The model under review builds one solid part; all positions refer to its coordinate system, in mm. Face numbers are marked on the shaded views. Round coordinates to 2 decimals unless told otherwise and drop trailing zeros. Loops run counter-clockwise (first coordinate to the right, second up) from the corner with the lowest first, then second, coordinate; pieces in that order, holes last. Notation, with made-up numbers: M -6.5,24 L 5.5,24 A12 ccw 5.5,46 Z; hole C -11,48 d5. An arc over 180 degrees is marked long. Answer as a JSON object with one key per item and string values. Group by question number.
Item 1: Consider section C-C (x = -20). Give the boundary of the cut face in (y, z), and give its area (3 significant figures).
Item 2: Consider section B-B (y = 2.7). Give the boundary of the cut face in (x, z).
Item 3: To check wall thickness, follow line 1 (X direction, y = 1.55, z = -6.35); line 2 (X direction, y = 1.6, z = -7); line 3 (Z direction, x = -5.5, y = 4.35). State the ranges of each line that lie inside material, in increasing order.
Item 4: The part is to be moulded in two halves that separate along X. For the marked faces 1, 2 and 3, say which applies: +X half, -X half, draft (parallel to the pull), parting line (faces both ways), or undercut.
Item 5: Insertion check: P1, Ø6, axis at x = -6.5, z = -5.5, coming from the -Y side. The pin has a flat end and moves straight along its axis. Give the tip position at first contact, or say it passes through.
Item 6: Consider section D-D (z = -8.25). Give the boundary of the cut face in (x, y), and give its area (3 significant figures).
Item 7: Consider section A-A (z = -6.35). Give the boundary of the cut face in (x, y), and give its area (3 significant figures).
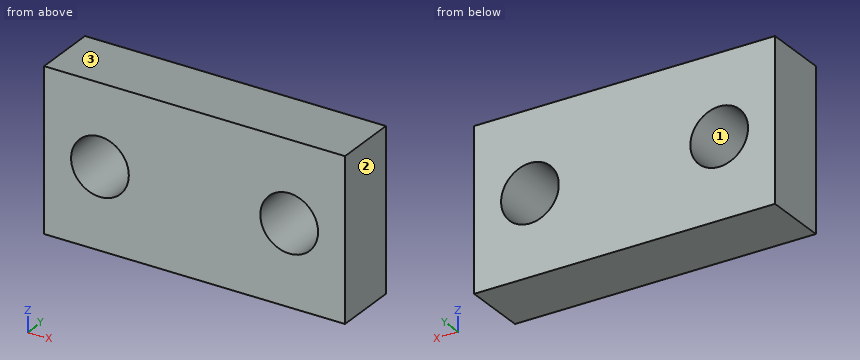
Autodesk Inventor part; units mm, degrees
ref_plane "YZ Plane" through (0, 0, 0) normal (1, 0, 0) x (0, 1, 0)
ref_plane "XZ Plane" through (0, 0, 0) normal (0, 1, 0) x (-1, 0, 0)
ref_plane "XY Plane" through (0, 0, 0) normal (0, 0, 1) x (1, 0, 0)
sketch "Spacer 2D" plane through (0, 0, 0) normal (0, 1, 0) x (-1, 0, 0)
  line L0 (12.4883, 0) -> (12.4883, -12.7) construction
  line L1 (24.4009, -12.7) -> (0.5757, -12.7)
  line L2 (0.5757, -12.7) -> (0.5757, 0)
  line L3 (0.5757, 0) -> (24.4009, 0)
  line L4 (24.4009, 0) -> (24.4009, -12.7)
  line L5 (24.4009, -12.7) -> (0.5757, 0) construction
  line L6 (0.5757, -12.7) -> (24.4009, 0) construction
  point P0 (0, 0)
  point P1 (12.4883, -6.35)
  dimension "d17" = 23.8252
  dimension "d18" = 12.7
extrude "Spacer Body" add sketch "Spacer 2D" along normal blind 5.08
sketch "Spacer Circles" plane through (0, 5.08, 0) normal (0, 1, 0) x (1, 0, 0)
  line L0 (-0.5757, 0) -> (-0.5757, 12.7) construction
  line L1 (-7.2813, 6.35) -> (-0.5757, 6.35) construction
  line L2 (-7.2813, 6.35) -> (-2.7093, 6.35) construction
  circle A0 centre (-4.9953, 6.35) radius 2.286
  line L3 (-17.6953, 6.35) -> (-7.2813, 6.35) construction
  line L4 (-17.6953, 6.35) -> (-24.4009, 6.35) construction
  line L5 (-24.4009, 12.7) -> (-24.4009, 0) construction
  line L6 (-0.5757, 0) -> (-24.4009, 0) construction
  line L7 (-24.4009, 0) -> (-24.4009, 12.7) construction
  line L8 (-24.4009, 12.7) -> (-0.5757, 12.7) construction
  line L9 (-0.5757, 12.7) -> (-0.5757, 0) construction
  line L10 (-12.4883, 6.35) -> (-12.4883, 0) construction
  line L11 (-24.4009, 0) -> (-0.5757, 0) construction
  circle A1 centre (-19.9813, 6.35) radius 2.286
  dimension "d25" = 4.572
  dimension "d26" = 10.414
  dimension "d31" = 2.1336
  dimension "d32" = 2.1336
extrude "Spacer Holes" cut sketch "Spacer Circles" against normal blind 10.16
properties part number "Rectangular Bottom Washer v1.2"
Geometry results:
{
 "1": {"outline": "M 0,-12.7 L 5.08,-12.7 L 5.08,-8.64 L 0,-8.64 Z; M 0,-4.06 L 5.08,-4.06 L 5.08,0 L 0,0 Z", "area": "41.3 mm^2"},
 "2": {"outline": "M -24.4,-12.7 L -0.58,-12.7 L -0.58,0 L -24.4,0 Z; hole C -19.98,-6.35 d4.57; hole C -5,-6.35 d4.57"},
 "3": {"line 1": "x = -24.4 to -22.27, -17.7 to -7.28, -2.71 to -0.58", "line 2": "x = -24.4 to -22.17, -17.79 to -7.19, -2.8 to -0.58", "line 3": "z = -12.7 to -8.58, -4.12 to 0"},
 "4": {"face 1": "undercut", "face 2": "+X half", "face 3": "draft"},
 "5": {"P1": "stops at y = 0"},
 "6": {"outline": "M -24.4,0 L -21.25,0 L -21.25,5.08 L -24.4,5.08 Z; M -18.71,0 L -6.27,0 L -6.27,5.08 L -18.71,5.08 Z; M -3.72,0 L -0.58,0 L -0.58,5.08 L -3.72,5.08 Z", "area": "95.2 mm^2"},
 "7": {"outline": "M -24.4,0 L -22.27,0 L -22.27,5.08 L -24.4,5.08 Z; M -17.7,0 L -7.28,0 L -7.28,5.08 L -17.7,5.08 Z; M -2.71,0 L -0.58,0 L -0.58,5.08 L -2.71,5.08 Z", "area": "74.6 mm^2"}
}
